Work out the finished part from the listing and answer in its coordinate system (mm). A direction names the side the tool comes from. Round coordinates to 2 decimals unless told otherwise and drop trailing zeros. Order: outer loops, then holes, each group sorted by start corner. A loop starts at its lowest first (then second) coordinate and runs counter-clockwise, first axis right, second up. Notation, with made-up numbers: M 55.5,36 L 85.5,36 A16 ccw 85.5,52 Z; hole C 21,-37 d9. An arc over 180 degrees is marked long. Answer as a JSON object with one key per item and string values. Group by question number.
Autodesk Inventor part; units mm, degrees
ref_plane "YZ Plane" through (0, 0, 0) normal (1, 0, 0) x (0, 1, 0)
ref_plane "XZ Plane" through (0, 0, 0) normal (0, 1, 0) x (-1, 0, 0)
ref_plane "XY Plane" through (0, 0, 0) normal (0, 0, 1) x (1, 0, 0)
sketch "Sketch1" plane through (0, 0, 0) normal (0, 1, 0) x (-1, 0, 0)
  circle A0 centre (0, 0) radius 72.5
  circle A1 centre (0, 0) radius 77.5
  circle A2 centre (0, 0) radius 53.5
  circle A3 centre (0, 0) radius 90 construction
  line L0 (0, 0) -> (-34.4415, 83.1492) construction
  circle A4 centre (-34.4415, 83.1492) radius 12
  line L1 (0, 154) -> (-32.5, 154)
  line L2 (-32.5, 154) -> (-32.5, 198)
  line L3 (-32.5, 198) -> (0, 198)
  line L4 (0, 198) -> (0, 154)
  line L5 (0, 140.825) -> (0, 198)
  line L6 (20, 74.8749) -> (-20, 74.8749)
  line L7 (-20, 74.8749) -> (-20, 154)
  line L8 (-20, 154) -> (20, 154)
  line L9 (20, 154) -> (20, 74.8749)
  line L10 (0, 0) -> (0, 198)
  line L11 (265, 193) -> (63.4449, 193)
  line L12 (63.4449, 193) -> (63.4449, 171)
  line L13 (63.4449, 171) -> (265, 171)
  line L14 (265, 171) -> (265, 193)
  line L15 (63.4449, 193) -> (0, 176)
  line L16 (63.4449, 171) -> (0, 154)
  line L17 (0, 154) -> (0, 176)
  arc A5 (-17.8117, 90.0375) -> (-51.0713, 76.2609) centre (-34.4415, 83.1492) ccw
  line L18 (-51.0713, 76.2609) -> (-45.4768, 62.7544)
  line L19 (-20, 74.8749) -> (-20, 106.132)
  line L20 (3.012, 3.8335) -> (-33.2222, -83.6438) construction
  line L21 (265, 182) -> (164.2224, 182)
  line L22 (164.2224, 182) -> (164.2224, 171)
  line L23 (164.2224, 171) -> (265, 171)
  line L24 (265, 171) -> (265, 182)
  line L25 (-17.8117, 90.0375) -> (-12.2171, 76.531)
  line L26 (-45.4768, 62.7544) -> (-12.2171, 76.531)
  point P0 (-41.2493, -65.6106)
  point P1 (-7.6728, -77.1192)
  dimension "oDiaGasket" = 145
  dimension "oDiaOutside" = 155
  dimension "oDiaInside" = 107
  dimension "oHoledia" = 24
  dimension "oStemThick" = 40
  dimension "oAngleFirstBolt" = 22.5
  dimension "oKcircle" = 180
  dimension "oDiaTop" = 65
  dimension "oHeightTop" = 44
  dimension "oHandleLenght" = 265
  dimension "d10" = 5
  dimension "d11" = 15
  dimension "d13" = 6
  dimension "oCenterTop" = 198
  dimension "d32" = 22.5
sketch "Sketch2" plane through (0, 0, 0) normal (0, 1, 0) x (-1, 0, 0)
  circle A0 centre (0, 0) radius 77.5
  circle A1 centre (0, 0) radius 53.5
  circle A2 centre (0, 0) radius 72.5
  circle A3 centre (0, 0) radius 53.5
  circle A4 centre (0, 0) radius 72.5
  circle A5 centre (0, 0) radius 77.5
extrude "Extrusion4" add sketch "Sketch2" along normal mid plane 56 contours A0 | A2
extrude "Extrusion5" add sketch "Sketch2" along normal mid plane 60 contours A2
extrude "Extrusion8" add sketch "Sketch1" along normal mid plane 56 contours A2 | L26 A1 L6 | L6 A1 L26 | L7 A5 L25 A1 | A1 L18 A5 L7 picked at (-33.064, 68.4842) picked at (-14.4207, 75.8246)
pattern_circular "Circular Pattern2" count 8 over 360 about axis through (0, 0, 0) along (0, 1, 0) of "Extrusion8"
extrude "Extrusion6" add sketch "Sketch1" along normal mid plane 40 contours A1 L10 L5 L8 L9 | A1 L25 A5 L7 L1 L5 L10 | L7 A5 L25 A1
revolve "Revolution1" add sketch "Sketch1" angle 360 about axis through (0, 0, 0) along (0, 0, 1) contours L1 L2 L3 L4
mirror "Mirror1" about plane through (0, 0, 0) normal (1, 0, 0) of "Extrusion8"
extrude "Extrusion9" add sketch "Sketch1" along normal mid plane 30 contours L4 L15 L12 L16 | L12 L11 L14 L21 L22 L13
chamfer "Chamfer1" distance 12 angle 45 4 edges at (-20, 20, 123.9468) (20, 20, 123.9468) (-20, -20, 123.9468) (20, -20, 123.9468)
equation "\"d32\" = oAngleFirstBolt"
equation "\"d25\" = oStemThick"
properties part number "BUTTERFLY VALVE MANUAL LUG TYPE DN100" material "GG25"
Item 1: Find section B-B (x = 0). Give the vertices of the cut face in (y, z), and give its area (3 significant figures).
Item 2: Find section A-A (z = 0). Give the vertices of the cut face in (x, y).
Item 3: Find section D-D (y = 0). Give the number of separate pieces and of enclosed holes in the cut face, and give its area (3 significant figures).
Item 4: Each of these flat-tipped pins is pushed along its axis until it touches: pin 1 (3 mm diameter, centred on x = -97, y = 13, fed in from +Z); pin 2 (24 mm diameter, centred on x = -198, y = -1.5, fed in from -Z); pin 3 (4 mm diameter, centred on x = 3.5, z = -68.5, fed in from +Y); pin 4 (12 mm diameter, centred on x = -26.5, z = 108.5, fed in from +Y). Where does it stop, or does it pass through?
Item 5: Consider L1, parallel to Z at x = 0, y = 29; L2, parallel to X at y = 18, z = 40.5; L3, parallel to Z at x = 75.5, y = -18. Determine where each line is inside the solid, lowest interval first.
Item 6: Find section C-C (z = 148). Give the vertices of the cut face in (x, y), and give its area (3 significant figures).
Item 7: The mould has two halves that part along X. Classify faces 1 (the flat face through (14, 15, 154)), 2 (the flat face through (-14, -14, 115)), 3 (the cylindrical face through (-69.15, -28.99, 21.78)), 4 (the flat face through (-83.379, -0.392, 15.054)): +X half, -X half, draft (parallel to the pull), parting line (faces both ways), or undercut.
Item 8: A tool of negligible diameter and unlimited length cuts with its end or side. For faces 5 (the flat face through (69.602, -0.392, 48.313)), 6 (the flat face through (5.7, -30, -53.4)), 7 (the flat face through (-15.054, -0.392, -83.379)), from which of +Z, -Z, +X, -X, +Y, -Y can it reach the whole face along a straight path? Write none if from no direction.
Responses:
{
 "1": {"outline": "M -32.5,154 L -20,154 L -20,77.5 L -28,77.5 L -28,72.5 L -30,72.5 L -30,53.5 L -28,53.5 L -28,-53.5 L -30,-53.5 L -30,-72.5 L -28,-72.5 L -28,-77.5 L 28,-77.5 L 28,-72.5 L 30,-72.5 L 30,-53.5 L 28,-53.5 L 28,53.5 L 30,53.5 L 30,72.5 L 28,72.5 L 28,77.5 L 20,77.5 L 20,154 L 32.5,154 L 32.5,198 L -32.5,198 Z", "area": "14,800 mm^2"},
 "2": {"outline": "M -77.5,-28 L -72.5,-28 L -72.5,-30 L -53.5,-30 L -53.5,-28 L 53.5,-28 L 53.5,-30 L 72.5,-30 L 72.5,-28 L 77.5,-28 L 77.5,28 L 72.5,28 L 72.5,30 L 53.5,30 L 53.5,28 L -53.5,28 L -53.5,30 L -72.5,30 L -72.5,28 L -77.5,28 Z"},
 "3": {"separate pieces": "1", "enclosed holes": "8", "area": "32,900 mm^2"},
 "4": {"pin 1": "stops at z = 193", "pin 2": "stops at z = 182", "pin 3": "stops at y = 30", "pin 4": "passes through"},
 "5": {"L1": "z = -72.5 to -53.5, 53.5 to 72.5, 154 to 198", "L2": "x = -100.1 to -93.51, -72.79 to 72.79, 93.51 to 100.1", "L3": "z = -50.76 to -43.69, -25.2 to 25.2, 43.69 to 50.76"},
 "6": {"outline": "M -20,-8 L -8,-20 L 8,-20 L 20,-8 L 20,8 L 8,20 L -8,20 L -20,8 Z", "area": "1,310 mm^2"},
 "7": {"face 1": "draft", "face 2": "undercut", "face 3": "parting line", "face 4": "-X half"},
 "8": {"face 5": "+Z, +Y, -Y", "face 6": "-Z, +X, -X, -Y", "face 7": "-Z, +Y, -Y"}
}
